Input: part model. Units: mm. Frame: model coordinates. Face numbers are marked on the shaded views. A direction names the side the tool comes from. Give positions to 0.01 mm unless a question says otherwise; leave off trailing zeros. Loops run counter-clockwise (first coordinate to the right, second up) from the corner with the lowest first, then second, coordinate; pieces in that order, holes last. Notation, with made-up numbers: (78.5, -9) -> (99.5, -9) arc R19 cw to (99.5, 18) -> close; hole circle Ø2 at (-33.75, -37). An arc over 180 degrees is marked (long way). One line per question, with ' | ' between items.
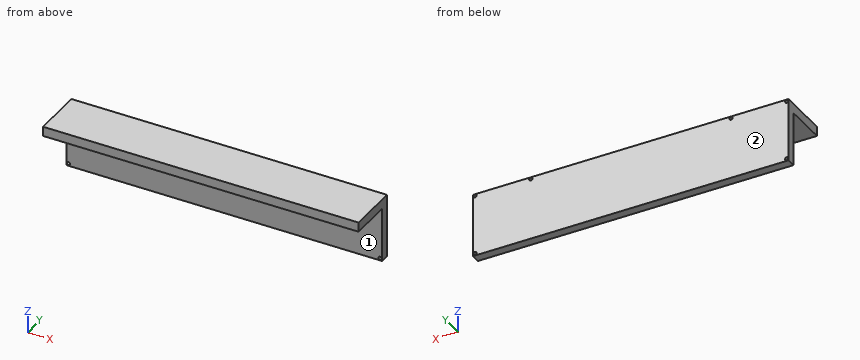
from build123d import *

# Parameters (mm, degrees)
F0_W     = 99
F0_H     = 3
F0_H_2   = 17
F1_DEPTH = 2.8
F2_DEPTH = 16
F3_R     = 0.5
F4_DEPTH = 3
F5_R     = 0.5
F6_DEPTH = 2.8
F7_DEPTH = 3


with BuildPart() as f1:
    # F0 (on Front) → F1 (new body)
    with BuildSketch(Plane.XZ):
        with Locations((-22.451522, 15.106464)):
            Rectangle(F0_W, F0_H)
        with Locations((-22.451522, 5.106464)):
            Rectangle(F0_W, F0_H_2)
    extrude(amount=F1_DEPTH)

    # F0 (on Front) → F2 (join)
    with BuildSketch(Plane.XZ):
        with Locations((-22.451522, 15.106464)):
            Rectangle(F0_W, F0_H)
    extrude(amount=F2_DEPTH)

    # F3 (on face) → F4 (cut)
    with BuildSketch(Plane.XZ):
        with Locations((26.443128, -2.697429)):
            Circle(F3_R)
        with Locations((-71.333528, -2.697429)):
            Circle(F3_R)
    extrude(amount=F4_DEPTH, mode=Mode.SUBTRACT)

    # F5 (on face) → F6 (cut)
    with BuildSketch(Plane.XZ):
        with Locations((26.413972, 16.001105)):
            Circle(F5_R)
        with Locations((-71.414955, 16.012859)):
            Circle(F5_R)
        with Locations((8.913972, 16.001105)):
            Circle(F5_R)
        with Locations((-53.914986, 16.045877)):
            Circle(F5_R)
    extrude(amount=F6_DEPTH, mode=Mode.SUBTRACT)

    # F5 (on face) → F7 (cut)
    with BuildSketch(Plane.XZ):
        with Locations((26.413972, 16.001105)):
            Circle(F5_R)
        with Locations((-71.414955, 16.012859)):
            Circle(F5_R)
        with Locations((8.913972, 16.001105)):
            Circle(F5_R)
        with Locations((-53.914986, 16.045877)):
            Circle(F5_R)
    extrude(amount=-F7_DEPTH, mode=Mode.SUBTRACT)


solid = f1.part
1. Ray query, line 1 along Z through (x, y) = (-14, -6.25); line 2 along Y through (x, z) = (2.5, 8.5). Return the intervals inside material, ascending. Write a range as from..to.
Determined:
line 1: z = 13.61..16.61 | line 2: y = -2.8..0
2. Reachability of the marked faces 1 and 2 from +Z, -Z, +X, -X, +Y, -Y: full face, straight path, thin tool, end or side. Return the list, or none.
Determined:
face 1: -Z, +X, -X, -Y | face 2: +Z, -Z, +X, -X, +Y
3. Section query A-A (y = -6.25). Output: boundary loops of the cut face in (x, z).
Determined:
outline: (-71.95, 13.61) -> (27.05, 13.61) -> (27.05, 16.61) -> (-71.95, 16.61) -> close
4. Section query C-C (z = 7). Output: boundary loops of the cut face in (x, y).
Determined:
outline: (-71.95, -2.8) -> (27.05, -2.8) -> (27.05, 0) -> (-71.95, 0) -> close
5. Section query B-B (x = -49.5). Output: boundary loops of the cut face in (y, z), then the cut area to 3 significant figures.
Determined:
outline: (-16, 13.61) -> (-2.8, 13.61) -> (-2.8, -3.39) -> (0, -3.39) -> (0, 16.61) -> (-16, 16.61) -> close | area: 95.6 mm2
6. Pin query (flat end, axial travel): P1, Ø1.5, axis at x = -0.5, z = 5.5, coming from the -Y side; P2, Ø6.5, axis at x = -31, y = -12.5, coming from the -Z side; P3, Ø0.5, axis at x = 9, z = 16, coming from the +Y side. Return the tip coordinate at first contact, or that it passes through.
Determined:
P1: stops at y = -2.8 | P2: stops at z = 13.61 | P3: stops at y = -2.8
